Can you work these out from the model? Positions are in its coordinate system, mm. A direction names the side the tool comes from. Give positions to 0.01 mm unless a question says otherwise; leave off trailing zeros. Write each loop counter-clockwise with the first axis right and the second up, starting at its lowest first coordinate (ties: lowest second). Pieces come first, ordered by that corner, then holes. Notation, with made-up numbers: (-34, 64) -> (-13, 64) arc R19 ccw to (-13, 81) -> close; hole circle Ø9 at (11, -25). An arc over 180 degrees is marked (long way). Answer as CSV lines item,"result". Start each with the question number.
1. If we section it at C-C on x = 109.5: Write out the boundary of the cut face in (y, z).
2. If we section it at B-B on y = 1.3: Count the separate pieces of the cut face and the enclosed holes in it, plus the area to 3 significant figures.
3. If we section it at A-A on z = -6.5: Write out the boundary of the cut face in (x, y).
4. I'm going to push flat-ended pins straight in: P1, Ø1.8, axis at x = -103, y = 3.5, coming from the -Z side; P2, Ø1.8, axis at x = -114, y = 3, coming from the +Z side. Where does each tip first touch, or does it pass through?
5. If we section it at D-D on z = -38.5: Write out the boundary of the cut face in (x, y), plus the area to 3 significant figures.
6. If we mould it in two halves opening along Z, with no side actions, what happens to faces 4 (the face through (-54, 3, 73.5)), 5 (the face through (-115, 3, -55)), 6 (the face through (140, 3, -73.5))? For each: pulls with the +Z half, pulls with the -Z half, needs draft (parallel to the pull), parting line crosses it, or undercut.
7. On a 3-axis mill with a long thin cutter (end or side, diameter ignored), from which of +Z, -Z, +X, -X, +Y, -Y can I reach the whole of each face in a straight line? I mean faces 1 (the face through (-108, 3, -67.5)), 2 (the face through (25, 3, 71)), 3 (the face through (-25, 3, -70)). Say none if no direction works.
8. I need wall thicknesses on line 1 (X direction, y = 2.25, z = 20); line 2 (X direction, y = 5.25, z = 28); line 3 (X direction, y = 4.1, z = -54). Which ranges of each line are inside material? Lowest first, please. Write a range as [from, to].
```python
from build123d import *

# Parameters (mm, degrees)
SALIENTE_EXTRUIR1_DEPTH = 6
CROQUIS2_W              = 58
CROQUIS2_H              = 6
SALIENTE_EXTRUIR2_DEPTH = 6
CROQUIS3_W              = 6
CROQUIS3_H              = 50
SALIENTE_EXTRUIR3_DEPTH = 6
CROQUIS5_W              = 5.95
CROQUIS5_H              = 110
CORTAR_EXTRUIR2_DEPTH   = 7
CROQUIS6_W              = 147
CROQUIS6_H              = 6
SALIENTE_EXTRUIR4_DEPTH = 14
CROQUIS7_W              = 5.95
CROQUIS7_H              = 95
CORTAR_EXTRUIR3_DEPTH   = 7


with BuildPart() as part:
    # Croquis1 → Saliente-Extruir1 (new body)
    with BuildSketch(Plane(origin=(0, 0, 0), x_dir=(1, 0, 0), z_dir=(0, 1, 0))):
        Polygon((-83, 67.5), (-133, 67.5), (-133, 25), (-133, -25), (-133, -67.5), (133, -67.5), (133, 67.5), (72.5, 67.5), (25, 67.5), (-25, 67.5), align=None)
    extrude(amount=SALIENTE_EXTRUIR1_DEPTH)

    # Croquis2 → Saliente-Extruir2 (add)
    with BuildSketch(Plane(origin=(0, 6, 0), x_dir=(1, 0, 0), z_dir=(0, 1, 0))):
        with Locations((-54, 70.5)):
            Rectangle(CROQUIS2_W, CROQUIS2_H)
        with Locations((54, 70.5)):
            Rectangle(CROQUIS2_W, CROQUIS2_H)
        with Locations((-54, -70.5)):
            Rectangle(CROQUIS2_W, CROQUIS2_H)
        with Locations((54, -70.5)):
            Rectangle(CROQUIS2_W, CROQUIS2_H)
    extrude(amount=-SALIENTE_EXTRUIR2_DEPTH)

    # Croquis3 → Saliente-Extruir3 (add)
    with BuildSketch(Plane(origin=(0, 6, 0), x_dir=(1, 0, 0), z_dir=(0, 1, 0))):
        with Locations((-136, 0)):
            Rectangle(CROQUIS3_W, CROQUIS3_H)
    extrude(amount=-SALIENTE_EXTRUIR3_DEPTH)

    # Croquis5 → Cortar-Extruir2 (cut, through all)
    with BuildSketch(Plane(origin=(0, 6, 0), x_dir=(1, 0, 0), z_dir=(0, 1, 0))):
        with Locations((-115.025, 0)):
            Rectangle(CROQUIS5_W, CROQUIS5_H)
    extrude(amount=-CORTAR_EXTRUIR2_DEPTH, mode=Mode.SUBTRACT)

    # Croquis6 → Saliente-Extruir4 (add)
    with BuildSketch(Plane(origin=(133, 0, 0), x_dir=(0, 0, -1), z_dir=(1, 0, 0))):
        with Locations((0, 3)):
            Rectangle(CROQUIS6_W, CROQUIS6_H)
    extrude(amount=SALIENTE_EXTRUIR4_DEPTH)

    # Croquis7 → Cortar-Extruir3 (cut, through all)
    with BuildSketch(Plane(origin=(0, 6, 0), x_dir=(1, 0, 0), z_dir=(0, 1, 0))):
        with Locations((140.025, 0)):
            Rectangle(CROQUIS7_W, CROQUIS7_H)
    extrude(amount=-CORTAR_EXTRUIR3_DEPTH, mode=Mode.SUBTRACT)


solid = part.part
```
Computed values:
1,outline,"(0, -67.5) -> (6, -67.5) -> (6, 67.5) -> (0, 67.5) -> close"
2,separate pieces,"1"
2,enclosed holes,"2"
2,area,"38,400 mm2"
3,outline,"(-139, 0) -> (-118, 0) -> (-118, 6) -> (-139, 6) -> close; (-112.05, 0) -> (137.05, 0) -> (137.05, 6) -> (-112.05, 6) -> close; (143, 0) -> (147, 0) -> (147, 6) -> (143, 6) -> close"
4,P1,"stops at z = -67.5"
4,P2,"stops at z = 67.5"
5,outline,"(-133, 0) -> (-118, 0) -> (-118, 6) -> (-133, 6) -> close; (-112.05, 0) -> (137.05, 0) -> (137.05, 6) -> (-112.05, 6) -> close; (143, 0) -> (147, 0) -> (147, 6) -> (143, 6) -> close"
5,area,"1,610 mm2"
6,face 4,"pulls with the +Z half"
6,face 5,"undercut"
6,face 6,"pulls with the -Z half"
7,face 1,"-Z, -X, +Y, -Y"
7,face 2,"+Z, +Y, -Y"
7,face 3,"-Z, +Y, -Y"
8,line 1,"x = [-139, -118], [-112.05, 137.05], [143, 147]"
8,line 2,"x = [-133, -118], [-112.05, 137.05], [143, 147]"
8,line 3,"x = [-133, -118], [-112.05, 147]"
